from build123d import *

# Parameters (mm, degrees)
SKETCH1_W               = 257.843094768
SKETCH1_H               = 107.95
BOSS_EXTRUDE1_DEPTH     = 6.35
SKETCH1_3_W             = 3.175
SKETCH1_3_H             = 90.678
BOSS_EXTRUDE2_DEPTH     = 19.05
SKETCH3_R               = 0.762
CUT_EXTRUDE1_DEPTH      = 6.35
SKETCH4_W               = 101.6
SKETCH4_H               = 101.6
CUT_EXTRUDE2_DEPTH      = 6.35
SKETCH5_W               = 130.944506092
SKETCH5_H               = 146.927254763
CUT_EXTRUDE3_DEPTH      = 35.56
CUT_EXTRUDE3_DEPTH_BACK = 45.974


with BuildPart() as part:
    # Sketch1 → Boss-Extrude1 (new body)
    with BuildSketch(Plane(origin=(0, 0, 0), x_dir=(1, 0, 0), z_dir=(0, 1, 0))):
        Rectangle(SKETCH1_W, SKETCH1_H)
    extrude(amount=-BOSS_EXTRUDE1_DEPTH)

    # Sketch1_3 → Boss-Extrude2 (add)
    with BuildSketch(Plane(origin=(0, 0, 0), x_dir=(1, 0, 0), z_dir=(0, 1, 0))):
        Polygon((-128.921547384, 53.975), (-128.921547384, 45.339), (-125.746547384, 45.339), (-122.571547384, 45.339), (-122.571547384, 53.975), align=None)
        Polygon((-96.917547384, 45.339), (-93.742547384, 45.339), (-93.742547384, 53.975), (-100.092547384, 53.975), (-100.092547384, 45.339), align=None)
        Polygon((-100.092547384, -45.339), (-100.092547384, -53.975), (-93.742547384, -53.975), (-93.742547384, -45.339), (-96.917547384, -45.339), align=None)
        Polygon((-128.921547384, -45.339), (-128.921547384, -53.975), (-122.571547384, -53.975), (-122.571547384, -45.339), (-125.746547384, -45.339), align=None)
        with Locations((-127.334047384, 0)):
            Rectangle(SKETCH1_3_W, SKETCH1_3_H)
        with Locations((-95.330047384, 0)):
            Rectangle(SKETCH1_3_W, SKETCH1_3_H)
    extrude(amount=BOSS_EXTRUDE2_DEPTH)

    # Sketch3 → Cut-Extrude1 (cut)
    with BuildSketch(Plane.XY.offset(53.975)):
        with Locations((-111.332047384, -1.651)):
            Circle(SKETCH3_R)
    cut_extrude1 = extrude(amount=-CUT_EXTRUDE1_DEPTH, mode=Mode.SUBTRACT)

    # Mirror1: Cut-Extrude1 across plane
    add(cut_extrude1.mirror(Plane.XY), mode=Mode.SUBTRACT)

    # Sketch4 → Cut-Extrude2 (cut)
    with BuildSketch(Plane(origin=(0, 0, 0), x_dir=(1, 0, 0), z_dir=(0, 1, 0))):
        with Locations((-33.003452616, 0)):
            Rectangle(SKETCH4_W, SKETCH4_H)
    extrude(amount=-CUT_EXTRUDE2_DEPTH, mode=Mode.SUBTRACT)

    # Sketch5 → Cut-Extrude3 (cut, two sides)
    with BuildSketch(Plane(origin=(0, 0, 0), x_dir=(1, 0, 0), z_dir=(0, 1, 0))) as cut_extrude3_sk:
        with Locations((-98.475705662, 18.035151403)):
            Rectangle(SKETCH5_W, SKETCH5_H)
    extrude(amount=CUT_EXTRUDE3_DEPTH, mode=Mode.SUBTRACT)
    extrude(cut_extrude3_sk.sketch, amount=-CUT_EXTRUDE3_DEPTH_BACK, mode=Mode.SUBTRACT)


solid = part.part
Can you work these out from the model? Positions are in its coordinate system, mm. A direction names the side the tool comes from. Coordinates: 2 decimals unless noted, no trailing zeros. Order: outer loops, then holes, each group sorted by start corner. A loop starts at its lowest first (then second) coordinate and runs counter-clockwise, first axis right, second up. Notation, with made-up numbers: (29, 15) - (49, 15) arc R34 ccw to (49, 45) - close; hole circle Ø11 at (35.25, -20). An arc over 180 degrees is marked (long way). Answer as a JSON object with one key per item and string values. Group by question number.
Q1. We'd pull the mould along Z, two halves only. Please class faces 3 (the face through (49, -3, -53.975)), 4 (the face through (47, -3, 53.975)), 5 (the face through (-8, -3, -50.8)), 6 (the face through (-33.003, -3, -52)): +Z half, -Z half, draft (parallel to the pull), parting line (faces both ways), or undercut.
Q2. Imagine slicing it at B-B (y = -4.5). Please give me the cut outline in (x, z) (3 decimals), and give its area (3 significant figures).
Q3. I need wall thicknesses on line 1 (Z direction, x = 0.5, y = -2.5) (3 decimals); line 2 (X direction, y = -1.5, z = 48). Which ranges of each line are inside material? Lowest first, please. Write a range as from..to.
Q4. On a 3-axis mill with a long thin cutter (end or side, diameter ignored), from which of +Z, -Z, +X, -X, +Y, -Y can I reach the whole of each face in a straight line? I mean faces 1 (the face through (-8, -3, 50.8)), 2 (the face through (-33.003, -3, 52)). Say none if no direction works.
Q5. Imagine slicing it at C-C (z = 1.5). Please give me the cut outline in (x, y).
Q6. Imagine slicing it at A-A (x = -4.5). Please give me the cut outline in (y, z) (3 decimals).
Q7. Will this pin go through, and if not, where does the flat tip stop? P1, Ø1.9, axis at y = -3, z = 16, coming from the -X side.
Determined:
{
 "1": {"face 3": "-Z half", "face 4": "+Z half", "face 5": "undercut", "face 6": "draft"},
 "2": {"outline": "(-33.003, -53.975) - (128.922, -53.975) - (128.922, 53.975) - (-33.003, 53.975) - (-33.003, 50.8) - (17.797, 50.8) - (17.797, -50.8) - (-33.003, -50.8) - close", "area": "12,300 mm2"},
 "3": {"line 1": "z = -53.975..-50.8, 50.8..53.975", "line 2": "x = 17.8..128.92"},
 "4": {"face 1": "-X, +Y, -Y", "face 2": "+Z, -Z, -X, +Y, -Y"},
 "5": {"outline": "(17.8, -6.35) - (128.92, -6.35) - (128.92, 0) - (17.8, 0) - close"},
 "6": {"outline": "(-6.35, -53.975) - (0, -53.975) - (0, -50.8) - (-6.35, -50.8) - close; (-6.35, 50.8) - (0, 50.8) - (0, 53.975) - (-6.35, 53.975) - close"},
 "7": {"P1": "stops at x = 17.8"}
}
